```python
from build123d import *

# Parameters (mm, degrees)
SK_DISC_R                 = 34
OUTPUT_DISC_DEPTH         = 6
SK_PILOT_R                = 22
PILOT_BOSS_DEPTH          = 2
SK_OUTHOLE_R              = 1.65
OUTPUT_TAPPED_HOLE_DEPTH  = 6
OUTPUT_HOLE_PATTERN_COUNT = 8


with BuildPart() as part:
    # SK_Disc → Output_Disc (new body)
    with BuildSketch(Plane.XY):
        Circle(SK_DISC_R)
    extrude(amount=OUTPUT_DISC_DEPTH)

    # SK_Pilot → Pilot_Boss (add)
    with BuildSketch(Plane.XY.offset(6)):
        Circle(SK_PILOT_R)
    extrude(amount=PILOT_BOSS_DEPTH)

    # SK_OutHole → Output_Tapped_Hole (cut)
    with BuildSketch(Plane.XY.offset(6)):
        with Locations((28, 0)):
            Circle(SK_OUTHOLE_R)
    output_tapped_hole = extrude(amount=-OUTPUT_TAPPED_HOLE_DEPTH, mode=Mode.SUBTRACT)

    # Output_Hole_Pattern: Output_Tapped_Hole ×8 about axis
    output_hole_pattern_axis = Axis((0, 0, 0), (0, 0, 1))
    for i in range(1, OUTPUT_HOLE_PATTERN_COUNT):
        add(output_tapped_hole.rotate(output_hole_pattern_axis, i * 360 / OUTPUT_HOLE_PATTERN_COUNT), mode=Mode.SUBTRACT)


solid = part.part
```
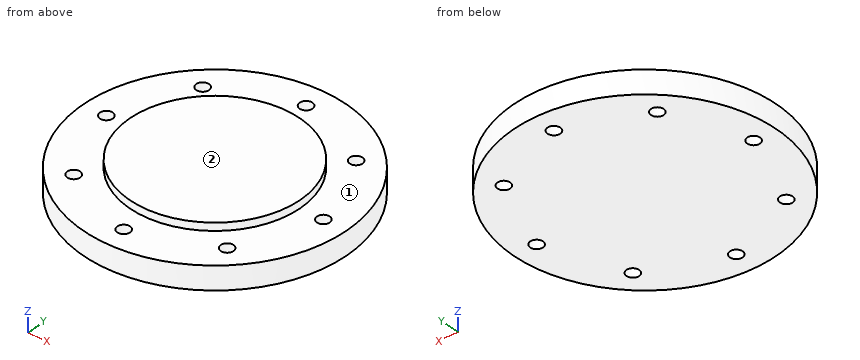
Geometry: final body of the model. Coordinates: model frame, mm. Face numbers are marked on the shaded views. A direction names the side the tool comes from. Coordinates: 2 decimals unless noted, no trailing zeros. Order: outer loops, then holes, each group sorted by start corner. A loop starts at its lowest first (then second) coordinate and runs counter-clockwise, first axis right, second up. Notation, with made-up numbers: (29, -23) -> (85, -23) arc R23 cw to (85, -1) -> close; hole circle Ø7 at (-22.75, 6.25). An arc over 180 degrees is marked (long way). Answer in a Markdown table with one row per item.
Item 1: Access query for the marked faces 1 and 2. Directions: +Z, -Z, +X, -X, +Y, -Y. A direction counts if a zero-diameter tool reaches every point of the face in a straight line with its end or side. Return the directions, or none.
Return value:
| item | result |
|---|---|
| face 1 | +Z |
| face 2 | +Z, +X, -X, +Y, -Y |
Item 2: Contact query for flat-ended pins moving along their axis: P1, Ø2.5, axis at x = 28, y = 0, coming from the +Z side; P2, Ø3, axis at x = 18.5, z = 5, coming from the +Y side; P3, Ø3, axis at x = -9.5, z = 4, coming from the -Y side; P4, Ø4, axis at x = -6, z = 5, coming from the -Y side. Output: stop coordinate, or through.
Return value:
| item | result |
|---|---|
| P1 | passes through |
| P2 | stops at y = 29.44 |
| P3 | stops at y = -33.05 |
| P4 | stops at y = -33.76 |
Item 3: Section B-B on y = -28. Output: boundary loops of the cut face in (x, z).
Return value:
| item | result |
|---|---|
| outline | (-19.29, 0) -> (-1.65, 0) -> (-1.65, 6) -> (-19.29, 6) -> close; (1.65, 0) -> (19.29, 0) -> (19.29, 6) -> (1.65, 6) -> close |
Item 4: Ray query, L1, parallel to Z at x = 17, y = -18; L2, parallel to X at y = 1, z = 4.5; L3, parallel to X at y = -8.5, z = 5.5. Return the intervals inside material, ascending.
Return value:
| item | result |
|---|---|
| L1 | z = 0 to 6 |
| L2 | x = -33.99 to -29.31, -26.69 to 26.69, 29.31 to 33.99 |
| L3 | x = -32.92 to 32.92 |
Item 5: Section D-D on z = 1.25. State how many separate pieces and enclosed holes the cut face has, plus the area to 3 significant figures.
Return value:
| item | result |
|---|---|
| separate pieces | 1 |
| enclosed holes | 8 |
| area | 3,560 mm² |
Item 6: Section A-A on x = 0. Output: boundary loops of the cut face in (y, z).
Return value:
| item | result |
|---|---|
| outline | (-34, 0) -> (-29.65, 0) -> (-29.65, 6) -> (-34, 6) -> close; (-26.35, 0) -> (26.35, 0) -> (26.35, 6) -> (22, 6) -> (22, 8) -> (-22, 8) -> (-22, 6) -> (-26.35, 6) -> close; (29.65, 0) -> (34, 0) -> (34, 6) -> (29.65, 6) -> close |
